```python
from build123d import *

# Parameters (mm, degrees)
F2_W     = 115
F2_H     = 25
F3_DEPTH = 1
F4_W     = 105
F4_H     = 16.148975119
F5_DEPTH = 9
F6_R     = 3.425
F7_DEPTH = 8


with BuildPart() as f3:
    # F2 (on Top) → F3 (new body)
    with BuildSketch(Plane.XY):
        Rectangle(F2_W, F2_H)
    extrude(amount=F3_DEPTH)

    # F4 (on face) → F5 (join)
    with BuildSketch(Plane.XY.offset(1)):
        Rectangle(F4_W, F4_H)
    extrude(amount=F5_DEPTH)

    # F6 (on face) → F7 (cut)
    with BuildSketch(Plane.XY.offset(10)):
        with Locations((-45, 0)):
            Circle(F6_R)
        with Locations((-30, 0)):
            Circle(F6_R)
        with Locations((-15, 0)):
            Circle(F6_R)
        Circle(F6_R)
        with Locations((15, 0)):
            Circle(F6_R)
        with Locations((30, 0)):
            Circle(F6_R)
        with Locations((45, 0)):
            Circle(F6_R)
    extrude(amount=-F7_DEPTH, mode=Mode.SUBTRACT)


solid = f3.part
```
CAD build for the part. Positions are in the model's coordinates, mm. A direction names the side the tool comes from. Round coordinates to 2 decimals unless told otherwise and drop trailing zeros. Order: outer loops, then holes, each group sorted by start corner. A loop starts at its lowest first (then second) coordinate and runs counter-clockwise, first axis right, second up.
Q1. Two-plate mould, pull along Y, no slides. Class faces 4 (the cylindrical face through (26.58, 0.15, 6.06)), 5 (the flat face through (-1, 4, 10)), 6 (the cylindrical face through (11.58, 0.15, 6.06)), 7 (the flat face through (-1, 8.074, 5)): pulls with the +Y half, pulls with the -Y half, needs draft (parallel to the pull), parting line crosses it, or undercut.
Q2. Slice it at A-A (z = 4.5). Write the cut outline in (x, y) (3 decimals), and give its area (3 significant figures).
Q3. Slice it at C-C (y = -6.5). Write the cut outline in (x, z), and give its area (3 significant figures).
Q4. Which spindle directions (+Z, -Z, +X, -X, +Y, -Y) get a long thin tool onto all of the face, cutting with end or side? Do faces 1 (the flat face through (-52.5, 0, 5)), 2 (the flat face through (-1, -8.074, 5)), 3 (the flat face through (45, 0, 2)). Say none if no direction does.
Q5. Drop flat-ended pins along their axis: pin 1 (2 mm diameter, centred on x = -16, y = 0, fed in from +Z); pin 2 (5 mm diameter, centred on y = 9, z = 5, fed in from +X); pin 3 (2.5 mm diameter, centred on x = -2.5, z = 7.5, fed in from -Y). Give the stop position or say it passes through.
Q6. Slice it at B-B (x = 21). Write the cut outline in (y, z).
Q7. Slice it at D-D (x = -45). Write the cut outline in (y, z) (3 decimals).
Q8. Wall check: L1, parallel to Y at x = 30, z = 7 (3 decimals); L2, parallel to X at y = 6.25, z = 2.5; L3, parallel to Y at x = 35, z = 2.5. Give the ranges that are in metal, low to high.
Results below:
1. face 4: undercut
1. face 5: needs draft
1. face 6: undercut
1. face 7: pulls with the +Y half
2. outline: (-52.5, -8.074) - (52.5, -8.074) - (52.5, 8.074) - (-52.5, 8.074) - close; hole circle Ø6.85 at (-45, 0); hole circle Ø6.85 at (-30, 0); hole circle Ø6.85 at (-15, 0); hole circle Ø6.85 at (0, 0); hole circle Ø6.85 at (15, 0); hole circle Ø6.85 at (30, 0); hole circle Ø6.85 at (45, 0)
2. area: 1,440 mm2
3. outline: (-57.5, 0) - (57.5, 0) - (57.5, 1) - (52.5, 1) - (52.5, 10) - (-52.5, 10) - (-52.5, 1) - (-57.5, 1) - close
3. area: 1,060 mm2
4. face 1: +Z, -X, +Y, -Y
4. face 2: +Z, +X, -X, -Y
4. face 3: +Z
5. pin 1: stops at z = 2
5. pin 2: stops at x = 52.5
5. pin 3: stops at y = -8.07
6. outline: (-12.5, 0) - (12.5, 0) - (12.5, 1) - (8.07, 1) - (8.07, 10) - (-8.07, 10) - (-8.07, 1) - (-12.5, 1) - close
7. outline: (-12.5, 0) - (12.5, 0) - (12.5, 1) - (8.074, 1) - (8.074, 10) - (3.425, 10) - (3.425, 2) - (-3.425, 2) - (-3.425, 10) - (-8.074, 10) - (-8.074, 1) - (-12.5, 1) - close
8. L1: y = -8.074 to -3.425, 3.425 to 8.074
8. L2: x = -52.5 to 52.5
8. L3: y = -8.07 to 8.07
